For this review, take the finished solid that the model builds, in its own axes (mm). Face numbers are marked on the shaded views. A direction names the side the tool comes from. Round coordinates to 2 decimals unless told otherwise and drop trailing zeros. Loops run counter-clockwise (first coordinate to the right, second up) from the corner with the lowest first, then second, coordinate; pieces in that order, holes last.
1) Take a section at D-D (y = 36.75). State the section outline as (x, z) points (3 decimals), then the cut area to 3 significant figures.
2) Wall thickness on L1, parallel to X at y = 31.5, z = -2.25; L2, parallel to Y at x = 14, z = -6.5; L3, parallel to X at y = 21.75, z = -1: over which ranges is each line inside the solid? List them lowest first.
3) Insertion check: pin 1 (6.5 mm diameter, centred on x = 5.35, z = 0, fed in from -Y); pin 2 (1 mm diameter, centred on x = 19, z = 10, fed in from +Y); pin 3 (2 mm diameter, centred on y = 24, z = 11, fed in from +X); pin 4 (1.5 mm diameter, centred on x = 5, y = 19, fed in from -Z). Each pin has a flat end and moves straight along its axis. Give the tip position at first contact, or say it passes through.
4) Tool access review of the marked faces 1 and 2: name each direction out of +Z, -Z, +X, -X, +Y, -Y from which nothing blocks a thin tool from reaching the whole face with its end or side.
5) Take a section at B-B (z = -3). State the section outline as (x, y) points.
6) Take a section at C-C (x = 16.5). State the section outline as (y, z) points.
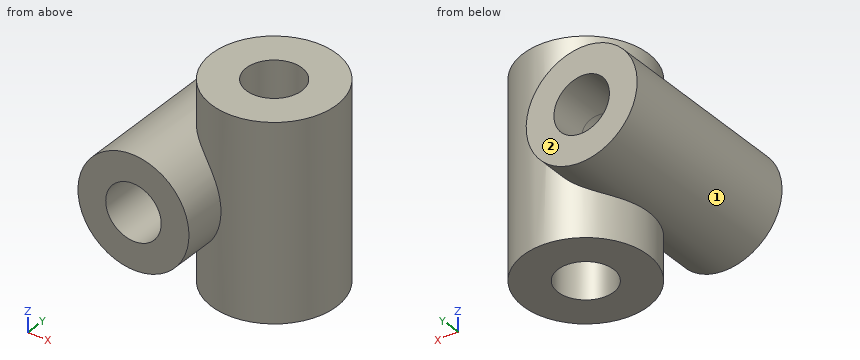
```python
from build123d import *

# Parameters (mm, degrees)
SKETCH1_R                = 16
SKETCH1_R_2              = 8
BOSS_EXTRUDE1_DEPTH      = 56
BOSS_EXTRUDE2_DEPTH      = 28
BOSS_EXTRUDE2_DEPTH_BACK = 28
SKETCH2_R                = 18
SKETCH2_R_2              = 8
SKETCH3_R                = 8
CUT_EXTRUDE1_DEPTH       = 73.221880507
SKETCH4_R                = 8
CUT_EXTRUDE2_DEPTH       = 87.994252854
ESCALA1_SCALE            = 0.5


with BuildPart() as part:
    # Sketch1 → Boss-Extrude1 (new body)
    with BuildSketch(Plane(origin=(0, 0, 0), x_dir=(1, 0, 0), z_dir=(0, 1, 0))):
        with Locations(Location((0, 0, 0), (0, 0, 270))):
            Circle(SKETCH1_R)
        with Locations(Location((0, 0, 0), (0, 0, 270))):
            Circle(SKETCH1_R_2, mode=Mode.SUBTRACT)
    extrude(amount=BOSS_EXTRUDE1_DEPTH)

    # Sketch2 → Boss-Extrude2 (add, two sides: drawn at the far end of the back side and taken through both)
    with BuildSketch(Plane.XY.offset(-BOSS_EXTRUDE2_DEPTH_BACK)):
        with Locations((18, 30.258098715)):
            Circle(SKETCH2_R)
        with Locations((18, 30.258098715)):
            Circle(SKETCH2_R_2, mode=Mode.SUBTRACT)
    extrude(amount=BOSS_EXTRUDE2_DEPTH + BOSS_EXTRUDE2_DEPTH_BACK)

    # Sketch3 → Cut-Extrude1 (cut, through all)
    with BuildSketch(Plane(origin=(0, 56, 0), x_dir=(1, 0, 0), z_dir=(0, 1, 0))):
        with Locations(Location((0, 0, 0), (0, 0, 270))):
            Circle(SKETCH3_R)
    extrude(amount=-CUT_EXTRUDE1_DEPTH, mode=Mode.SUBTRACT)

    # Sketch4 → Cut-Extrude2 (cut, through all)
    with BuildSketch(Plane.XY.offset(28)):
        with Locations((18, 30.258098715)):
            Circle(SKETCH4_R)
    extrude(amount=-CUT_EXTRUDE2_DEPTH, mode=Mode.SUBTRACT)


with BuildPart() as part_1:
    # Escala1: scaled about (10.696977917, 29.156321687, 4.4659e-05)
    add(part.part.scale(ESCALA1_SCALE).moved(Location((5.348488958, 14.578160843, 2.233e-05))))


solid = part_1.part
```
Response:
1. outline: (8.745, -14) - (19.952, -14) - (19.952, 14) - (8.745, 14) - (8.745, 7.243) arc R8 ccw (long way) to (8.745, -7.243) - close; hole circle Ø8 at (5.348, 0)
1. area: 417 mm2
2. L1: x = -2.33 to 2.04, 8.66 to 10.77, 17.92 to 23.17
2. L2: y = 20.71 to 25.72, 33.69 to 38.7
2. L3: x = -2.59 to 1.48, 9.22 to 18.55
3. pin 1: passes through
3. pin 2: stops at y = 37.69
3. pin 3: stops at x = 22.02
3. pin 4: stops at z = -8
4. face 1: none
4. face 2: +Z, -Z, +X, -X, +Y
5. outline: (-2.07, 14.58) - (2.7, 14.58) - (2.7, 42.58) - (-2.07, 42.58) - close; (7.99, 14.58) - (12.76, 14.58) - (12.76, 20.85) arc R9 ccw (long way) to (12.76, 38.57) - (12.76, 42.58) - (7.99, 42.58) - close; hole circle Ø8 at (14.35, 29.71)
6. outline: (20.97, -14) - (26.34, -14) - (26.34, 14) - (20.97, 14) - close; (33.08, -14) - (38.45, -14) - (38.45, 14) - (33.08, 14) - close
